Source: CAD feature listing. Evaluate the final solid. Frame: model axes, mm. Face numbers are marked on the shaded views. A direction names the side the tool comes from. Coordinates: 2 decimals unless noted, no trailing zeros. Loops run counter-clockwise (first coordinate to the right, second up) from the corner with the lowest first, then second, coordinate; pieces in that order, holes last.
from build123d import *

# Parameters (mm, degrees)
SKETCH1_R             = 32.5
SKETCH1_R_2           = 2
BOSS_EXTRUDE1_DEPTH   = 9.5
CUT_EXTRUDE1_DEPTH    = 3.5
BOSS_EXTRUDE2_START   = 4
SKETCH4_R             = 17.5
BOSS_EXTRUDE2_DEPTH   = 4
BOSS_EXTRUDE4_START   = 17.5
SKETCH5_R             = 10
BOSS_EXTRUDE4_DEPTH   = 17.5
SKETCH6_R             = 1.225
CUT_EXTRUDE2_DEPTH    = 20
F_4_0MM_DOWEL_HOLE1_D = 4
CIRPATTERN1_COUNT     = 4
FILLET1_R             = 1


with BuildPart() as part:
    # Sketch1 → Boss-Extrude1 (new body)
    with BuildSketch(Plane.XY):
        Circle(SKETCH1_R)
        with Locations((0, 28)):
            Circle(SKETCH1_R_2, mode=Mode.SUBTRACT)
        with Locations((12, 24.2)):
            Circle(SKETCH1_R_2, mode=Mode.SUBTRACT)
        with Locations((-12, 24.2)):
            Circle(SKETCH1_R_2, mode=Mode.SUBTRACT)
        with Locations((-12, -24.2)):
            Circle(SKETCH1_R_2, mode=Mode.SUBTRACT)
        with Locations((0, -28)):
            Circle(SKETCH1_R_2, mode=Mode.SUBTRACT)
        with Locations((12, -24.2)):
            Circle(SKETCH1_R_2, mode=Mode.SUBTRACT)
        with BuildLine():
            Line((-1, 3.872983346), (-1, 5.002983346))
            Line((-1, 5.002983346), (1, 5.002983346))
            Line((1, 5.002983346), (1, 3.872983346))
            ThreePointArc((1, 3.872983346), (0, -4), (-1, 3.872983346))
        make_face(mode=Mode.SUBTRACT)
    extrude(amount=BOSS_EXTRUDE1_DEPTH)

    # Sketch2 → Cut-Extrude1 (cut)
    with BuildSketch(Plane(origin=(0, 0, 0), x_dir=(-1, 0, 0), z_dir=(0, 0, -1))):
        with BuildLine():
            ThreePointArc((-14.609747332, 21.50709843), (-26, 0), (-14.609747332, -21.50709843))
            ThreePointArc((-14.609747332, -21.50709843), (-13.665935552, -27.559636697), (-8.276785753, -24.647409957))
            ThreePointArc((-8.276785753, -24.647409957), (-5.252947534, -25.463828114), (-2.152878353, -25.910714286))
            ThreePointArc((-2.152878353, -25.910714286), (0, -31), (2.152878353, -25.910714286))
            ThreePointArc((2.152878353, -25.910714286), (5.252947534, -25.463828114), (8.276785753, -24.647409957))
            ThreePointArc((8.276785753, -24.647409957), (13.665935552, -27.559636697), (14.609747332, -21.50709843))
            ThreePointArc((14.609747332, -21.50709843), (26, 0), (14.609747332, 21.50709843))
            ThreePointArc((14.609747332, 21.50709843), (13.665935552, 27.559636697), (8.276785753, 24.647409957))
            ThreePointArc((8.276785753, 24.647409957), (5.252947534, 25.463828114), (2.152878353, 25.910714286))
            ThreePointArc((2.152878353, 25.910714286), (0, 31), (-2.152878353, 25.910714286))
            ThreePointArc((-2.152878353, 25.910714286), (-5.252947534, 25.463828114), (-8.276785753, 24.647409957))
            ThreePointArc((-8.276785753, 24.647409957), (-13.665935552, 27.559636697), (-14.609747332, 21.50709843))
        make_face()
    extrude(amount=-CUT_EXTRUDE1_DEPTH, mode=Mode.SUBTRACT)

    # Sketch4 → Boss-Extrude2 (add)
    with BuildSketch(Plane(origin=(0, 0, 3.5), x_dir=(-1, 0, 0), z_dir=(0, 0, -1)).offset(BOSS_EXTRUDE2_START)):
        Circle(SKETCH4_R)
        with BuildLine():
            Line((1, 5.002983346), (1, 3.872983346))
            ThreePointArc((1, 3.872983346), (0, -4), (-1, 3.872983346))
            Line((-1, 3.872983346), (-1, 5.002983346))
            Line((-1, 5.002983346), (1, 5.002983346))
        make_face(mode=Mode.SUBTRACT)
    extrude(amount=-BOSS_EXTRUDE2_DEPTH)

    # Sketch5 → Boss-Extrude4 (add)
    with BuildSketch(Plane(origin=(0, 0, -0.5), x_dir=(-1, 0, 0), z_dir=(0, 0, -1)).offset(BOSS_EXTRUDE4_START)):
        Circle(SKETCH5_R)
        with BuildLine():
            Line((-1, 5.002983346), (-1, 3.872983346))
            ThreePointArc((-1, 3.872983346), (0, -4), (1, 3.872983346))
            Line((1, 3.872983346), (1, 5.002983346))
            Line((1, 5.002983346), (-1, 5.002983346))
        make_face(mode=Mode.SUBTRACT)
    extrude(amount=-BOSS_EXTRUDE4_DEPTH)

    # Sketch6 → Cut-Extrude2 (cut, symmetric)
    with BuildSketch(Plane(origin=(0, 0, 0), x_dir=(0, 0, -1), z_dir=(1, 0, 0))):
        with Locations((6.8, 0)):
            Circle(SKETCH6_R)
    extrude(amount=CUT_EXTRUDE2_DEPTH, both=True, mode=Mode.SUBTRACT)

    # Ø4.0mm Dowel Hole1 (through all)
    with Locations(Plane(origin=(0, 0, -18), x_dir=(-1, 0, 0), z_dir=(0, 0, -1))):
        with Locations((5, 5)):
            f_4_0mm_dowel_hole1 = Hole(F_4_0MM_DOWEL_HOLE1_D / 2)

    # CirPattern1: Ø4.0mm Dowel Hole1 ×4 about axis
    cirpattern1_axis = Axis((0, 0, 0), (0, 0, 1))
    for i in range(1, CIRPATTERN1_COUNT):
        add(f_4_0mm_dowel_hole1.rotate(cirpattern1_axis, i * 360 / CIRPATTERN1_COUNT), mode=Mode.SUBTRACT)

    # Fillet1
    fillet1_edges = [part.edges().sort_by_distance(p)[0] for p in [
        (10, 0, -0.5),
    ]]
    fillet(fillet1_edges, radius=FILLET1_R)


solid = part.part
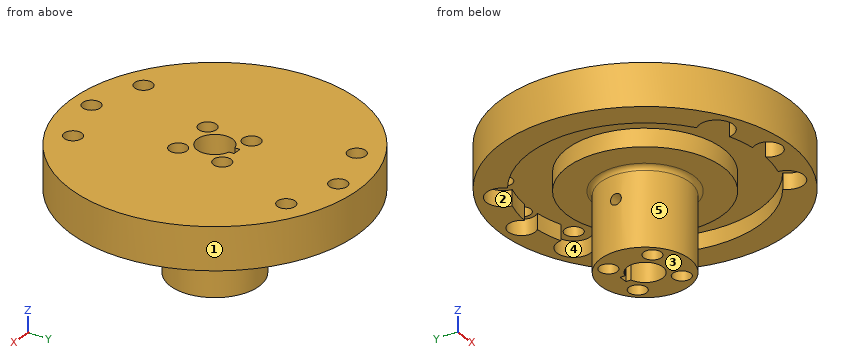
Q1. Section A-A, the plane z = 5.5. Count the separate pieces of the cut face and the enclosed holes in it, plus the area to 3 significant figures.
Q2. Draft query along X for the marked faces 3, 4 and 5. Return one class per face: +X half, -X half, draft (parallel to the pull), parting line (faces both ways), or undercut.
Q3. Section C-C, the plane z = -11.5. Return the cut outline in (x, y).
Q4. Section B-B, the plane x = 12. Return the cut outline in (y, z), plus the area to 3 significant figures.
Q5. Section D-D, the plane y = -20. Return the cut outline in (x, z).
Q6. Access query for the marked faces 1 and 2. Directions: +Z, -Z, +X, -X, +Y, -Y. A direction counts if a zero-diameter tool reaches every point of the face in a straight line with its end or side. Return the directions, or none.
Q7. Line query: line 1 along Y through (x, z) = (4.5, -10.5); line 2 along X through (y, z) = (24.2, 5.35); line 3 along Z through (x, y) = (-5, 0) (3 decimals). Output: solid intervals per line, ascending.
Q8. Contact query for flat-ended pins moving along their axis: pin 1 Ø8.5 at (x, y) = (12, 24.2) entering from -Z; pin 2 Ø6.5 at (x, y) = (0, 0) entering from +Z; pin 3 Ø2 at (x, z) = (0.5, -4.5) entering from -Y; pin 4 Ø5 at (x, z) = (-24, 2) entering from +Y. Output: stop coordinate, or through.
Derived:
1. separate pieces: 1
1. enclosed holes: 11
1. area: 3,140 mm2
2. face 3: draft
2. face 4: undercut
2. face 5: parting line
3. outline: circle Ø20 at (0, 0); hole circle Ø4 at (-5, -5); hole circle Ø4 at (-5, 5); hole (-1, 3.87) arc R4 ccw (long way) to (1, 3.87) - (1, 5) - (-1, 5) - close; hole circle Ø4 at (5, -5); hole circle Ø4 at (5, 5)
4. outline: (-30.2, 0) - (-27.95, 0) - (-27.95, 3.5) - (-26.2, 3.5) - (-26.2, 9.5) - (-30.2, 9.5) - close; (-22.2, 3.5) - (-12.74, 3.5) - (-12.74, -0.5) - (12.74, -0.5) - (12.74, 3.5) - (22.2, 3.5) - (22.2, 9.5) - (-22.2, 9.5) - close; (26.2, 3.5) - (27.95, 3.5) - (27.95, 0) - (30.2, 0) - (30.2, 9.5) - (26.2, 9.5) - close
4. area: 432 mm2
5. outline: (-25.62, 0) - (-16.61, 0) - (-16.61, 3.5) - (16.61, 3.5) - (16.61, 0) - (25.62, 0) - (25.62, 9.5) - (-25.62, 9.5) - close
6. face 1: +Z, -Z
6. face 2: -Z
7. line 1: y = -8.93 to -6.94, -3.06 to 3.06, 6.94 to 8.93
7. line 2: x = -21.69 to -14, -10 to 10, 14 to 21.69
7. line 3: z = -18 to -8.025, -5.575 to 9.5
8. pin 1: stops at z = 0
8. pin 2: passes through
8. pin 3: stops at y = -10
8. pin 4: stops at y = 24.37
